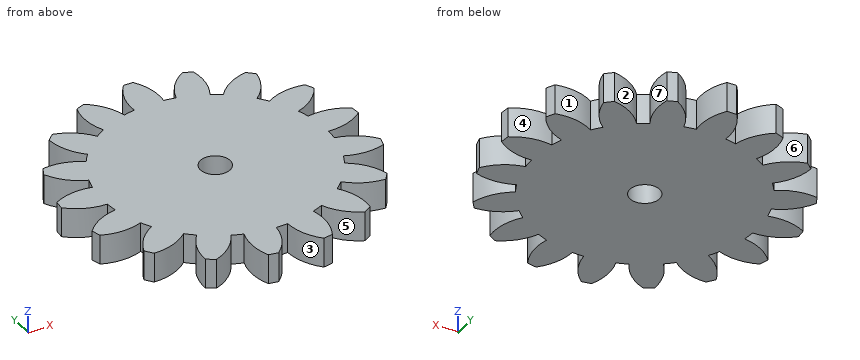
from build123d import *

# Parameters (mm, degrees)
SKIZZE1_R                       = 20
AUFSATZ_LINEAR_AUSTRAGEN1_DEPTH = 4
SCHNITT_LINEAR_AUSTRAGEN1_REACH = 6
SKIZZE2_R                       = 2
SCHNITT_LINEAR_AUSTRAGEN2_DEPTH = 4
KREISMUSTER1_COUNT              = 17


with BuildPart() as part:
    # Skizze1 → Aufsatz-Linear austragen1 (new body)
    with BuildSketch(Plane.XY):
        Circle(SKIZZE1_R)
    extrude(amount=AUFSATZ_LINEAR_AUSTRAGEN1_DEPTH)

    # Skizze2 → Schnitt-Linear austragen1 (cut, up to next)
    with BuildSketch(Plane.XY.offset(4), mode=Mode.PRIVATE) as schnitt_linear_austragen1_sk1:
        Circle(SKIZZE2_R)
    schnitt_linear_austragen1_tool1 = extrude(schnitt_linear_austragen1_sk1.sketch, amount=-SCHNITT_LINEAR_AUSTRAGEN1_REACH, mode=Mode.PRIVATE) & part.part
    add(schnitt_linear_austragen1_tool1.solids().sort_by_distance((0, 0, 4))[0], mode=Mode.SUBTRACT)

    # Skizze3 → Schnitt-Linear austragen2 (cut)
    with BuildSketch(Plane.XY.offset(4)):
        with BuildLine():
            ThreePointArc((0.586774522, 19.991390538), (1.647430818, 17.553771601), (1.751244892, 14.897420627))
            ThreePointArc((1.751244892, 14.897420627), (2.516627793, 14.787379232), (3.275322949, 14.638041521))
            ThreePointArc((3.275322949, 14.638041521), (4.506718961, 17.083727504), (6.562201755, 18.892789845))
            ThreePointArc((6.562201755, 18.892789845), (3.616448026, 19.670315292), (0.586774522, 19.991390538))
        make_face()
    schnitt_linear_austragen2 = extrude(amount=-SCHNITT_LINEAR_AUSTRAGEN2_DEPTH, mode=Mode.SUBTRACT)

    # Kreismuster1: Schnitt-Linear austragen2 ×17 about axis
    kreismuster1_axis = Axis((0, 0, 0), (0, 0, 1))
    for i in range(1, KREISMUSTER1_COUNT):
        add(schnitt_linear_austragen2.rotate(kreismuster1_axis, i * 360 / KREISMUSTER1_COUNT), mode=Mode.SUBTRACT)


solid = part.part
Geometry: final body of the model. Coordinates: model frame, mm. Face numbers are marked on the shaded views. A direction names the side the tool comes from. Round coordinates to 2 decimals unless told otherwise and drop trailing zeros. Write each loop counter-clockwise with the first axis right and the second up, starting at its lowest first coordinate (ties: lowest second). Pieces come first, ordered by that corner, then holes. Notation, with made-up numbers: M -22,-31.75 L -4,-31.75 A7 cw -4,-20.75 Z; hole C 39.5,44 d8. An arc over 180 degrees is marked long. Write item = value, one per line.
Item 1: Pin query (flat end, axial travel): P1, Ø2, axis at y = -13, z = 3.5, coming from the +X side; P2, Ø2, axis at x = -5, z = 2, coming from the -Y side. Return the tip coordinate at first contact, or that it passes through.
Findings:
P1 = 16
P2 = -19.6
Item 2: Access query for the marked faces 1, 2 and 3. Directions: +Z, -Z, +X, -X, +Y, -Y. A direction counts if a zero-diameter tool reaches every point of the face in a straight line with its end or side. Return the directions, or none.
Findings:
face_1 = +Z, -Z
face_2 = +Z, -Z, +Y
face_3 = +Z, -Z, -Y
Item 3: Pull-direction query (Y, two-part tool) for the marked faces 4, 5, 6 and 7; classes: pulls with the +Y half, pulls with the -Y half, needs draft (parallel to the pull), parting line crosses it, or undercut.
Findings:
face_4 = undercut
face_5 = pulls with the -Y half
face_6 = pulls with the +Y half
face_7 = undercut
Item 4: Section query A-A on x = 0. Return loops of the section in (y, z).
Findings:
outline = M -15,0 L -2,0 L -2,4 L -15,4 Z; M 2,0 L 20,0 L 20,4 L 2,4 Z
Item 5: Material intervals for line 1 along Y through (x, z) = (0, 3.2); line 2 along Y through (x, z) = (17, 3.55); line 3 along X through (y, z) = (-11, 1.5), sorted ascending. Write a range as [from, to].
Findings:
line_1 = [-15, -2], [2, 20]
line_2 = [-6.4, -2.66], [-0.2, 3.63], [6.85, 9.64]
line_3 = [-16.08, -10.81], [-10.2, 10.2], [11.53, 16.23]
Item 6: Section query B-B on y = 0.5. Return loops of the section in (x, z).
Findings:
outline = M -19.2,0 L -1.94,0 L -1.94,4 L -19.2,4 Z; M 1.94,0 L 18.83,0 L 18.83,4 L 1.94,4 Z
Item 7: Section query C-C on y = -8.5. Return loops of the section in (x, z), then the cut area to 3 significant figures.
Findings:
outline = M -14.26,0 L 14.78,0 L 14.78,4 L -14.26,4 Z
area = 116 mm^2
